Can you work these out from the model? Positions are in its coordinate system, mm. Face numbers are marked on the shaded views. A direction names the side the tool comes from. Round coordinates to 2 decimals unless told otherwise and drop trailing zeros. Write each loop counter-clockwise with the first axis right and the second up, starting at its lowest first coordinate (ties: lowest second). Pieces come first, ordered by that corner, then holes. Notation, with made-up numbers: M 83.25,73.5 L 100.25,73.5 A20 ccw 100.25,82.5 Z; hole C -3,71.5 d3. An arc over 180 degrees is marked long. Answer as a JSON object with one key per item and string values. Group by question number.
1) I'm going to push flat-ended pins straight in: pin 1 Ø2 at (x, z) = (23, -4.5) entering from -Y; pin 2 Ø1.5 at (y, z) = (2.5, -4) entering from +X; pin 3 Ø1.5 at (x, z) = (70.5, 2.5) entering from +Y. Where does each tip first touch, or does it pass through?
2) Suppose I cut it at D-D, the plane z = 4. Write out the boundary of the cut face in (x, y), and give its area (3 significant figures).
3) If we mould it in two halves opening along Y, with no side actions, what happens to the marked faces 3, 4 and 5? For each: +Y half, -Y half, draft (parallel to the pull), parting line (faces both ways), or undercut.
4) Suppose I cut it at C-C, the plane x = 53. Write out the boundary of the cut face in (y, z).
5) Please list where these lines run through material, in increasing order: L1, parallel to X at y = 0, z = 0 (1 decimal); L2, parallel to X at y = 0, z = -3.25; L3, parallel to X at y = -2.5, z = -2. Write a range as [from, to].
6) On a 3-axis mill with a long thin cutter (end or side, diameter ignored), from which of +Z, -Z, +X, -X, +Y, -Y can I reach the whole of each face in a straight line? I mean the marked faces 1 and 2. Say none if no direction works.
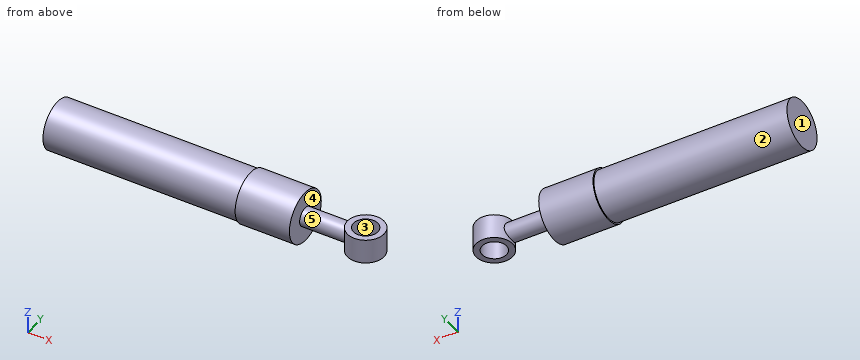
from build123d import *

# Parameters (mm, degrees)
SKETCH3_R           = 4.7625
SKETCH3_R_2         = 3.175
BOSS_EXTRUDE1_DEPTH = 3.175


with BuildPart() as part:
    # Sketch2 → Revolve1 (revolve)
    with BuildSketch(Plane.XY):
        Polygon((0, 0), (0, 6.35), (50.8, 6.35), (50.8, 6.7183), (65.0875, 6.7183), (65.0875, 2.413), (77.7875, 2.413), (77.7875, 0), align=None)
    revolve(axis=Axis((0, 0, 0), (1, 0, 0)))

    # Sketch3 → Boss-Extrude1 (add, symmetric)
    with BuildSketch(Plane.XY):
        with Locations((80.9625, 0)):
            Circle(SKETCH3_R)
        with Locations((80.9625, 0)):
            Circle(SKETCH3_R_2, mode=Mode.SUBTRACT)
    extrude(amount=BOSS_EXTRUDE1_DEPTH, both=True)


solid = part.part
Results:
{
 "1": {"pin 1": "y = -5.3", "pin 2": "x = 65.09", "pin 3": "y = 1.66"},
 "2": {"outline": "M 0,-4.93 L 50.8,-4.93 L 50.8,-5.4 L 65.09,-5.4 L 65.09,5.4 L 50.8,5.4 L 50.8,4.93 L 0,4.93 Z", "area": "655 mm^2"},
 "3": {"face 3": "undercut", "face 4": "draft", "face 5": "parting line"},
 "4": {"outline": "C 0,0 d13.44"},
 "5": {"L1": "[0, 77.8], [84.1, 85.7]", "L2": "[0, 65.09]", "L3": "[0, 65.09], [76.91, 79.01], [82.92, 85.02]"},
 "6": {"face 1": "+Z, -Z, -X, +Y, -Y", "face 2": "-X"}
}
